```python
from build123d import *

# Parameters (mm, degrees)
SKETCH1_W           = 45
SKETCH1_H           = 40
BOSS_EXTRUDE1_DEPTH = 6
SKETCH2_W           = 5
SKETCH2_H           = 5
SKETCH2_H_2         = 7
CUT_EXTRUDE1_DEPTH  = 6
SKETCH3_W           = 5
SKETCH3_H           = 5
SKETCH3_H_2         = 3
SKETCH3_H_3         = 10
CUT_EXTRUDE2_DEPTH  = 6
SKETCH4_W           = 5
SKETCH4_H           = 7
CUT_EXTRUDE3_DEPTH  = 6


with BuildPart() as part:
    # Sketch1 → Boss-Extrude1 (new body)
    with BuildSketch(Plane.XY):
        with Locations((1.238898757, -2.615452931)):
            Rectangle(SKETCH1_W, SKETCH1_H)
    extrude(amount=BOSS_EXTRUDE1_DEPTH)

    # Sketch2 → Cut-Extrude1 (cut)
    with BuildSketch(Plane.XY.offset(6)):
        with Locations((-18.761101243, 4.884547069)):
            Rectangle(SKETCH2_W, SKETCH2_H)
        with Locations((-18.761101243, -4.115452931)):
            Rectangle(SKETCH2_W, SKETCH2_H_2)
        with Locations((-18.761101243, -15.115452931)):
            Rectangle(SKETCH2_W, SKETCH2_H)
    extrude(amount=-CUT_EXTRUDE1_DEPTH, mode=Mode.SUBTRACT)

    # Sketch3 → Cut-Extrude2 (cut)
    with BuildSketch(Plane.XY.offset(6)):
        with Locations((21.238898757, -20.115452931)):
            Rectangle(SKETCH3_W, SKETCH3_H)
        with Locations((21.238898757, -9.115452931)):
            Rectangle(SKETCH3_W, SKETCH3_H_2)
        with Locations((21.238898757, 14.884547069)):
            Rectangle(SKETCH3_W, SKETCH3_H)
        with Locations((21.238898757, 2.384547069)):
            Rectangle(SKETCH3_W, SKETCH3_H_3)
    extrude(amount=-CUT_EXTRUDE2_DEPTH, mode=Mode.SUBTRACT)

    # Sketch4 → Cut-Extrude3 (cut)
    with BuildSketch(Plane.XY.offset(6)):
        with Locations((21.238898757, -19.115452931)):
            Rectangle(SKETCH4_W, SKETCH4_H)
    extrude(amount=-CUT_EXTRUDE3_DEPTH, mode=Mode.SUBTRACT)


solid = part.part
```
The model under review builds one solid part; all positions refer to its coordinate system, in mm. A direction names the side the tool comes from. Give positions to 0.01 mm unless a question says otherwise; leave off trailing zeros. Write each loop counter-clockwise with the first axis right and the second up, starting at its lowest first coordinate (ties: lowest second). Pieces come first, ordered by that corner, then holes. Notation, with made-up numbers: (34, 43.25) -> (51, 43.25) arc R16 ccw to (51, 59.25) -> close; hole circle Ø1 at (68, 43). An arc over 180 degrees is marked (long way). Put each result on its own line as item: value.
(1) To check wall thickness, follow probe 1 along X at (y, z) = (-17.5, 2.2); probe 2 along X at (y, z) = (14.5, 4.55). State the ranges of each line that lie inside material, in increasing order. Write a range as from..to.
Results are:
probe 1: -16.26..18.74
probe 2: -21.26..18.74
(2) We need section A-A, the plane z = 0.7. Give the boundary of the cut face in (x, y).
Results are:
outline: (-21.26, -22.62) -> (18.74, -22.62) -> (18.74, -15.62) -> (23.74, -15.62) -> (23.74, -10.62) -> (18.74, -10.62) -> (18.74, -7.62) -> (23.74, -7.62) -> (23.74, -2.62) -> (18.74, -2.62) -> (18.74, 7.38) -> (23.74, 7.38) -> (23.74, 12.38) -> (18.74, 12.38) -> (18.74, 17.38) -> (-21.26, 17.38) -> (-21.26, 7.38) -> (-16.26, 7.38) -> (-16.26, 2.38) -> (-21.26, 2.38) -> (-21.26, -0.62) -> (-16.26, -0.62) -> (-16.26, -7.62) -> (-21.26, -7.62) -> (-21.26, -12.62) -> (-16.26, -12.62) -> (-16.26, -17.62) -> (-21.26, -17.62) -> close
(3) The part is to be moulded in two halves that separate along Y. For faces 1 (the flat face through (21, 7.385, 3)), 2 (the flat face through (23.739, -13, 3)), 3 (the flat face through (21, 12.385, 3)), say which applies: pulls with the +Y half, pulls with the -Y half, needs draft (parallel to the pull), parting line crosses it, or undercut.
Results are:
face 1: undercut
face 2: needs draft
face 3: pulls with the +Y half
(4) Tool access review of faces 4 (the flat face through (18.739, 2, 3)), 5 (the flat face through (1, -2, 0)), 6 (the flat face through (18.739, 15, 3)), 7 (the flat face through (-16.261, -15, 3)): name each direction out of +Z, -Z, +X, -X, +Y, -Y from which nothing blocks a thin tool from reaching the whole face with its end or side.
Results are:
face 4: +Z, -Z, +X
face 5: -Z, +X, -X, +Y, -Y
face 6: +Z, -Z, +X, +Y
face 7: +Z, -Z, -X
(5) We need section C-C, the plane y = -5. Give the boundary of the cut face in (x, z), and give its area (3 significant figures).
Results are:
outline: (-16.26, 0) -> (23.74, 0) -> (23.74, 6) -> (-16.26, 6) -> close
area: 240 mm²
(6) For pin 1 Ø1.5 at (x, z) = (21, 3.5) entering from +Y; pin 2 Ø3 at (y, z) = (-4, 3.5) entering from -X; pin 3 Ø2.5 at (x, z) = (20.5, 3.5) entering from -Y, all flat-tipped, find the tip position at first contact; note any pin that passes through.
Results are:
pin 1: y = 12.38
pin 2: x = -16.26
pin 3: y = -15.62
(7) We need section B-B, the plane y = 5. Give the boundary of the cut face in (x, z), and give its area (3 significant figures).
Results are:
outline: (-16.26, 0) -> (18.74, 0) -> (18.74, 6) -> (-16.26, 6) -> close
area: 210 mm²
